For this review, take the finished solid that the model builds, in its own axes (mm). A direction names the side the tool comes from. Coordinates: 2 decimals unless noted, no trailing zeros. Loops run counter-clockwise (first coordinate to the right, second up) from the corner with the lowest first, then second, coordinate; pieces in that order, holes last.
```python
from build123d import *

# Parameters (mm, degrees)
F1_DEPTH      = 10
F1_DEPTH_BACK = 10
F2_SIZE       = 4
F4_D          = 4
F4_DEPTH      = 10
F4_TIP        = 1.2017212381
F6_D          = 12
F6_DEPTH      = 17
F6_TIP        = 3.6051637142


with BuildPart() as f1:
    # F0 (on Front) → F1 (new body, two sides)
    with BuildSketch(Plane.XZ) as f1_sk:
        Polygon((-14, 40), (-14, -40), (14, -40), (14, -10), (29, -10), (29, 10), (14, 10), (14, 40), align=None)
        with BuildLine():
            ThreePointArc((-5, 27), (0, 32), (5, 27))
            Line((5, 27), (5, -27))
            ThreePointArc((5, -27), (0, -32), (-5, -27))
            Line((-5, -27), (-5, 27))
        make_face(mode=Mode.SUBTRACT)
    extrude(amount=F1_DEPTH)
    extrude(f1_sk.sketch, amount=-F1_DEPTH_BACK)

    # F2
    f2_edges = [f1.edges().sort_by_distance(p)[0] for p in [
        (14, 0, 40),
        (-14, 0, 40),
        (14, 0, -40),
        (-14, 0, -40),
    ]]
    chamfer(f2_edges, length=F2_SIZE)

    # F4
    with Locations(Plane.XZ.offset(10)):
        with Locations((23, 0)):
            Hole(F4_D / 2, depth=F4_DEPTH)
            with Locations((0, 0, -(F4_DEPTH + F4_TIP / 2))):  # 118° drill point
                Cone(0, F4_D / 2, F4_TIP, mode=Mode.SUBTRACT)

    # F6
    with Locations(Plane.YZ.offset(29)):
        with Locations((0, 0)):
            Hole(F6_D / 2, depth=F6_DEPTH)
            with Locations((0, 0, -(F6_DEPTH + F6_TIP / 2))):  # 118° drill point
                Cone(0, F6_D / 2, F6_TIP, mode=Mode.SUBTRACT)


solid = f1.part
```
Q1. For pin 1 Ø5 at (x, y) = (21.5, 5.5) entering from +Z; pin 2 Ø1.5 at (y, z) = (-2, -30) entering from +X; pin 3 Ø8 at (x, z) = (0.5, 1.5) entering from +Y; pin 4 Ø12 at (x, y) = (19.5, 5) entering from +Z, all flat-tipped, find the tip position at first contact; note any pin that passes through.
Q2. Consider section A-A (z = 24.5). State the section outline as (x, y) points, then the cut area to 3 significant figures.
Q3. Consider section C-C (y = -7.25). State the section outline as (x, z) points, then the cut area to 3 significant figures.
Q4. Consider section B-B (x = 0). State the section outline as (y, z) points, then the cut area to 3 significant figures.
Q5. The part is to be moulded in two halves that separate along Y. For faces 5 (the face through (7, -10, 1)), 6 (the face through (23, -8, 2)), 7 (the face through (20.38, 4.76, -3.65)), 8 (the face through (9.02, 0.48, -0.92)), say which applies: +Y half, -Y half, draft (parallel to the pull), parting line (faces both ways), or undercut.
Q6. Wall thickness on probe 1 along X at (y, z) = (-6.95, 0); probe 2 along Z at (x, y) = (23, -8.4); probe 3 along X at (y, z) = (2.5, -8): over which ranges is each line inside the solid? List them lowest first.
Q7. Consider section D-D (x = 23). State the section outline as (y, z) points.
Q8. Machinability: for faces 1 (the face through (14, 0, 23)), 2 (the face through (0, 0, 32)), 3 (the face through (0, 0, 40)), 4 (the face through (21, 0, -10)), which of the approach directions +Z, -Z, +X, -X, +Y, -Y give a long, thin tool a straight path to every point of the face, cutting with its end or side? Answer none if there is none.
Model answer:
1. pin 1: stops at z = 10
1. pin 2: stops at x = 14
1. pin 3: passes through
1. pin 4: stops at z = 36.5
2. outline: (-14, -10) - (-5, -10) - (-5, 10) - (-14, 10) - close; (5, -10) - (14, -10) - (14, 10) - (5, 10) - close
2. area: 360 mm2
3. outline: (-14, -36) - (-10, -40) - (10, -40) - (14, -36) - (14, -10) - (29, -10) - (29, 10) - (14, 10) - (14, 36) - (10, 40) - (-10, 40) - (-14, 36) - close; hole (-5, -27) arc R5 ccw to (5, -27) - (5, 27) arc R5 ccw to (-5, 27) - close; hole circle Ø4 at (23, 0)
3. area: 1,880 mm2
4. outline: (-10, -40) - (10, -40) - (10, -32) - (-10, -32) - close; (-10, 32) - (10, 32) - (10, 40) - (-10, 40) - close
4. area: 320 mm2
5. face 5: -Y half
5. face 6: draft
5. face 7: undercut
5. face 8: undercut
6. probe 1: x = -14 to -5, 5 to 21, 25 to 29
6. probe 2: z = -10 to -2, 2 to 10
6. probe 3: x = -14 to -5, 5 to 29
7. outline: (-10, -10) - (10, -10) - (10, 10) - (-10, 10) - (-10, 2) - (-5.66, 2) arc R6 cw (long way) to (-5.66, -2) - (-10, -2) - close
8. face 1: +Z, +X, +Y, -Y
8. face 2: +Y, -Y
8. face 3: +Z, +X, -X, +Y, -Y
8. face 4: -Z, +X, +Y, -Y
